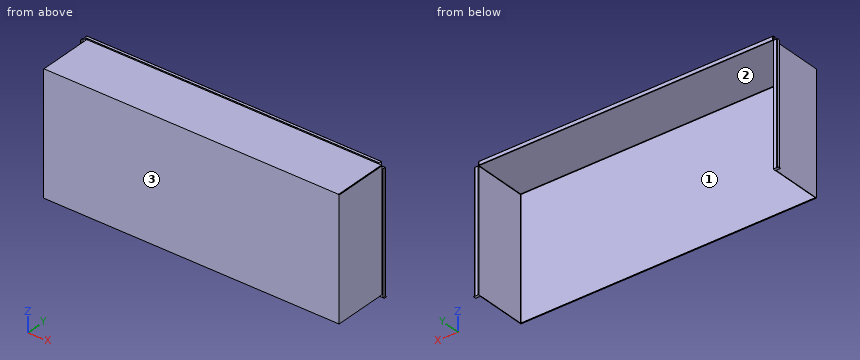
```python
from build123d import *

# Parameters (mm, degrees)
BOSS_EXTRUDE1_DEPTH = 336.55
SKETCH2_W           = 14.2875
SKETCH2_H           = 7.9375
BOSS_EXTRUDE2_DEPTH = 0.508
BOSS_EXTRUDE6_DEPTH = 412.7627
FILLET1_R           = 1.016
FILLET2_R           = 1.016
FILLET3_R           = 1.016
FILLET4_R           = 1.016
FILLET5_R           = 1.016


with BuildPart() as part:
    # Sketch1 → Boss-Extrude1 (new body)
    with BuildSketch(Plane.XY):
        Polygon((-412.75, 0), (412.75, 0), (412.75, 149.225), (423.8625, 149.225), (423.8625, 141.2875), (423.3545, 141.2875), (423.3545, 148.717), (414.3375, 148.717), (414.3375, -3.175), (-414.3375, -3.175), (-414.3375, 148.717), (-423.3545, 148.717), (-423.3545, 141.2875), (-423.8625, 141.2875), (-423.8625, 149.225), (-412.75, 149.225), align=None)
    extrude(amount=BOSS_EXTRUDE1_DEPTH)

    # Sketch2 → Boss-Extrude2 (add)
    with BuildSketch(Plane(origin=(0, 0, 0), x_dir=(-1, 0, 0), z_dir=(0, 0, -1))):
        with Locations((-419.89375, 145.25625)):
            Rectangle(SKETCH2_W, SKETCH2_H)
        with Locations((419.89375, 145.25625)):
            Rectangle(SKETCH2_W, SKETCH2_H)
    extrude(amount=BOSS_EXTRUDE2_DEPTH)

    # Sketch3 → Boss-Extrude6 (add, symmetric)
    with BuildSketch(Plane(origin=(0, 0, 0), x_dir=(0, 0, -1), z_dir=(1, 0, 0))):
        Polygon((-336.55, -3.175), (-336.55, 149.225), (-347.6625, 149.225), (-347.6625, 141.2875), (-347.1545, 141.2875), (-347.1545, 148.717), (-338.1375, 148.717), (-338.1375, -3.175), align=None)
    extrude(amount=BOSS_EXTRUDE6_DEPTH, both=True)

    # Fillet1
    fillet1_edges = [part.edges().sort_by_distance(p)[0] for p in [
        (412.75, 74.6125, 336.55),
    ]]
    fillet(fillet1_edges, radius=FILLET1_R)

    # Fillet2
    fillet2_edges = [part.edges().sort_by_distance(p)[0] for p in [
        (412.7627, 73.025, 336.55),
    ]]
    fillet(fillet2_edges, radius=FILLET2_R)

    # Fillet3
    fillet3_edges = [part.edges().sort_by_distance(p)[0] for p in [
        (-412.75, 74.6125, 336.55),
        (-412.7627, 73.025, 336.55),
    ]]
    fillet(fillet3_edges, radius=FILLET3_R)

    # Fillet4
    fillet4_edges = [part.edges().sort_by_distance(p)[0] for p in [
        (0, 0, 336.55),
        (412.75, 0, 167.767),
        (412.45242049, 0, 336.25242049),
        (-412.75, 0, 167.767),
        (-412.45242049, 0, 336.25242049),
    ]]
    fillet(fillet4_edges, radius=FILLET4_R)

    # Fillet5
    # the kernel refuses this fillet: 1.016 mm, written as the material it takes off along each edge
    with BuildSketch(Plane(origin=(413.7787, 149.225, 336.55), x_dir=(0, 0, -1), z_dir=(1, 0, 0)), Plane(origin=(-426.4025, 149.225, 336.55), x_dir=(0, 0, -1), z_dir=(1, 0, 0))) as fillet5_piece_1:
        with BuildLine():
            CenterArc((FILLET5_R, -FILLET5_R), FILLET5_R, 90, 90)
            Line((0, -FILLET5_R), (0, 0))
            Line((0, 0), (FILLET5_R, 0))
        make_face()
    fillet5_piece_1_solid = extrude(amount=12.6238, mode=Mode.PRIVATE)
    with BuildSketch(Plane(origin=(413.7787, 149.225, 337.566), x_dir=(0, 0, -1), z_dir=(1, 0, 0))) as fillet5_piece_2:
        with BuildLine():
            CenterArc((1.016 + FILLET5_R, -FILLET5_R), FILLET5_R, 90, 90)
            Line((1.016, -FILLET5_R), (1.016, 0))
            Line((1.016, 0), (1.016 + FILLET5_R, 0))
        make_face()
    fillet5_piece_2_solid = revolve(axis=Axis((413.7787, 149.225, 337.566), (0, 1, 0)), revolution_arc=90, mode=Mode.PRIVATE)
    with BuildSketch(Plane(origin=(-413.7787, 149.225, 337.566), x_dir=(1, 0, 0), z_dir=(0, 0, 1))) as fillet5_piece_3:
        with BuildLine():
            CenterArc((1.016 + FILLET5_R, -FILLET5_R), FILLET5_R, 90, 90)
            Line((1.016, -FILLET5_R), (1.016, 0))
            Line((1.016, 0), (1.016 + FILLET5_R, 0))
        make_face()
    fillet5_piece_3_solid = revolve(axis=Axis((-413.7787, 149.225, 337.566), (0, 1, 0)), revolution_arc=90, mode=Mode.PRIVATE)
    with BuildSketch(Plane(origin=(-412.75, 149.225, -3.048), x_dir=(0, -1, 0), z_dir=(0, 0, 1))) as fillet5_piece_4:
        with BuildLine():
            CenterArc((FILLET5_R, -FILLET5_R), FILLET5_R, 90, 90)
            Line((0, -FILLET5_R), (0, 0))
            Line((0, 0), (FILLET5_R, 0))
        make_face()
    fillet5_piece_4_solid = extrude(amount=338.582, mode=Mode.PRIVATE)
    with BuildSketch(Plane(origin=(-411.734, 149.225, 335.534), x_dir=(0, 0, 1), z_dir=(1, 0, 0))) as fillet5_piece_5:
        with BuildLine():
            CenterArc((1.016 + FILLET5_R, FILLET5_R), FILLET5_R, 180, 90)
            Line((1.016 + FILLET5_R, 0), (1.016, 0))
            Line((1.016, 0), (1.016, FILLET5_R))
        make_face()
    fillet5_piece_5_solid = revolve(axis=Axis((-411.734, 149.225, 335.534), (0, -1, 0)), revolution_arc=90, mode=Mode.PRIVATE)
    with BuildSketch(Plane(origin=(-411.734, 149.225, 336.55), x_dir=(0, 0, 1), z_dir=(1, 0, 0))) as fillet5_piece_6:
        with BuildLine():
            CenterArc((FILLET5_R, FILLET5_R), FILLET5_R, 180, 90)
            Line((0, FILLET5_R), (0, 0))
            Line((0, 0), (FILLET5_R, 0))
        make_face()
    fillet5_piece_6_solid = extrude(amount=823.468, mode=Mode.PRIVATE)
    with BuildSketch(Plane(origin=(411.734, 149.225, 335.534), x_dir=(1, 0, 0), z_dir=(0, 0, -1))) as fillet5_piece_7:
        with BuildLine():
            CenterArc((1.016 + FILLET5_R, FILLET5_R), FILLET5_R, 180, 90)
            Line((1.016, FILLET5_R), (1.016, 0))
            Line((1.016, 0), (1.016 + FILLET5_R, 0))
        make_face()
    fillet5_piece_7_solid = revolve(axis=Axis((411.734, 149.225, 335.534), (0, -1, 0)), revolution_arc=90, mode=Mode.PRIVATE)
    with BuildSketch(Plane(origin=(412.7627, 149.225, 337.566), x_dir=(-1, 0, 0), z_dir=(0, 0, 1))) as fillet5_piece_8:
        with BuildLine():
            CenterArc((FILLET5_R, FILLET5_R), FILLET5_R, 180, 90)
            Line((0, FILLET5_R), (0, 0))
            Line((0, 0), (FILLET5_R, 0))
        make_face()
    fillet5_piece_8_solid = extrude(amount=12.6365, mode=Mode.PRIVATE)
    with BuildSketch(Plane(origin=(-412.7627, 149.225, 337.566), x_dir=(1, 0, 0), z_dir=(0, 0, 1))) as fillet5_piece_9:
        with BuildLine():
            CenterArc((FILLET5_R, -FILLET5_R), FILLET5_R, 90, 90)
            Line((0, -FILLET5_R), (0, 0))
            Line((0, 0), (FILLET5_R, 0))
        make_face()
    fillet5_piece_9_solid = extrude(amount=12.6365, mode=Mode.PRIVATE)
    with BuildSketch(Plane(origin=(-415.3027, 149.225, 347.6625), x_dir=(0, 0, -1), z_dir=(1, 0, 0))) as fillet5_piece_10:
        with BuildLine():
            CenterArc((FILLET5_R, -FILLET5_R), FILLET5_R, 90, 90)
            Line((0, -FILLET5_R), (0, 0))
            Line((0, 0), (FILLET5_R, 0))
        make_face()
    fillet5_piece_10_solid = extrude(amount=830.6054, mode=Mode.PRIVATE)
    with BuildSketch(Plane(origin=(-423.8625, 149.225, 0), x_dir=(1, 0, 0), z_dir=(0, 0, 1))) as fillet5_piece_11:
        with BuildLine():
            CenterArc((FILLET5_R, -FILLET5_R), FILLET5_R, 90, 90)
            Line((0, -FILLET5_R), (0, 0))
            Line((0, 0), (FILLET5_R, 0))
        make_face()
    fillet5_piece_11_solid = extrude(amount=339.09, mode=Mode.PRIVATE)
    with BuildSketch(Plane(origin=(412.75, 149.225, 335.534), x_dir=(1, 0, 0), z_dir=(0, 0, -1))) as fillet5_piece_12:
        with BuildLine():
            CenterArc((FILLET5_R, FILLET5_R), FILLET5_R, 180, 90)
            Line((0, FILLET5_R), (0, 0))
            Line((0, 0), (FILLET5_R, 0))
        make_face()
    fillet5_piece_12_solid = extrude(amount=338.582, mode=Mode.PRIVATE)
    with BuildSketch(Plane(origin=(423.8625, 149.225, 0), x_dir=(-1, 0, 0), z_dir=(0, 0, 1))) as fillet5_piece_13:
        with BuildLine():
            CenterArc((FILLET5_R, FILLET5_R), FILLET5_R, 180, 90)
            Line((0, FILLET5_R), (0, 0))
            Line((0, 0), (FILLET5_R, 0))
        make_face()
    fillet5_piece_13_solid = extrude(amount=339.09, mode=Mode.PRIVATE)
    add([fillet5_piece_1_solid, fillet5_piece_2_solid, fillet5_piece_3_solid, fillet5_piece_4_solid, fillet5_piece_5_solid, fillet5_piece_6_solid, fillet5_piece_7_solid, fillet5_piece_8_solid, fillet5_piece_9_solid, fillet5_piece_10_solid, fillet5_piece_11_solid, fillet5_piece_12_solid, fillet5_piece_13_solid], mode=Mode.SUBTRACT)


solid = part.part
```
Verification items for the finished model (mm, model axes). Face numbers are marked on the shaded views. Give positions to 0.01 mm unless a question says otherwise; leave off trailing zeros. Loops run counter-clockwise (first coordinate to the right, second up) from the corner with the lowest first, then second, coordinate; pieces in that order, holes last.
1. Section check B-B, the plane y = 23.5. Enter the section's corners in (x, z).
2. Go/stop test with flat-tipped pins: pin 1 Ø4.5 at (x, z) = (418, 113.5) entering from -Y; pin 2 Ø5 at (x, y) = (-142, 116) entering from +Z; pin 3 Ø3.5 at (x, y) = (-424, 146.5) entering from +Z. Record where each tip stops, or that it passes through.
3. Thickness scan on line 1 (X direction, y = 111.5, z = 188); line 2 (Y direction, x = 81, z = 242.5) (3 decimals). Record the ranges inside material, lowest first.
4. Mould release check, pull along X, two halves, no side actions. Record for the marked faces 1, 2 and 3: released by +X, released by -X, zero draft, split by the parting line, or undercut.
Geometry says:
1. outline: (-414.34, 0) - (-412.75, 0) - (-412.75, 335.53) arc R1.02 cw to (-411.73, 336.55) - (411.73, 336.55) arc R1.02 cw to (412.75, 335.53) - (412.75, 0) - (414.34, 0) - (414.34, 336.55) - (413.78, 336.55) arc R1.02 cw to (412.76, 337.57) - (412.76, 338.14) - (-412.76, 338.14) - (-412.76, 337.57) arc R1.02 cw to (-413.78, 336.55) - (-414.34, 336.55) - close
2. pin 1: stops at y = 148.72
2. pin 2: stops at z = 338.14
2. pin 3: stops at z = 336.55
3. line 1: x = -414.34 to -412.75, 412.75 to 414.34
3. line 2: y = -3.175 to 0
4. face 1: undercut
4. face 2: undercut
4. face 3: zero draft
